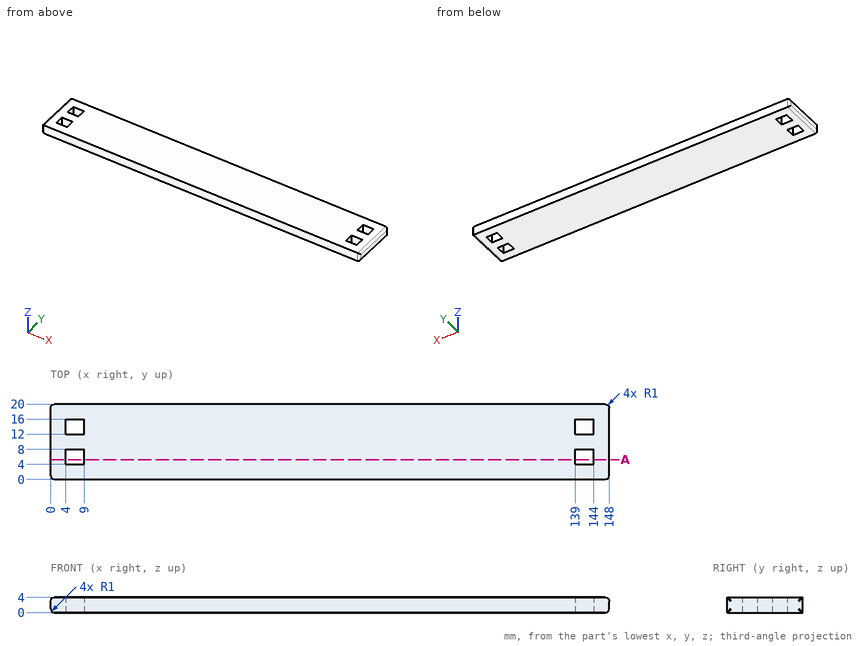
Can you work these out from the drawing? Everything is in mm from the part's minimum corner. Coordinates: 2 decimals unless noted, no trailing zeros. Loops run counter-clockwise (first coordinate to the right, second up) from the corner with the lowest first, then second, coordinate; pieces in that order, holes last. Notation, with made-up numbers: M 63,25 L 91,25 A32 ccw 91,59 Z; hole C -4.5,87.25 d8. An arc over 180 degrees is marked long. Put each result on its own line as item: value. Start each with the question number.
(1) I need wall thicknesses on line 1 (X direction, y = 4.75, z = 2.65); line 2 (Y direction, x = 6.5, z = 0.75); line 3 (X direction, y = 7.5, z = 0.6). Which ranges of each line are inside material? Lowest first, please. Write a range as from..to.
(2) Will this pin go through, and if not, where does the flat tip stop? P1, Ø1.2, axis at y = 6, z = 2, coming from the -X side.
(3) Suppose I cut it at A-A on y = 5.25. Please give me the cut outline in (x, z).
Solutions:
1. line 1: x = 0..4, 9..139, 144..148
1. line 2: y = 0..4, 8..12, 16..20
1. line 3: x = 0.08..4, 9..139, 144..147.92
2. P1: stops at x = 0
3. outline: M 0,1 A1 ccw 1,0 L 4,0 L 4,4 L 1,4 A1 ccw 0,3 Z; M 9,0 L 139,0 L 139,4 L 9,4 Z; M 144,0 L 147,0 A1 ccw 148,1 L 148,3 A1 ccw 147,4 L 144,4 Z
